Source: CAD feature listing. Evaluate the final solid. Frame: model axes, mm. Coordinates: 2 decimals unless noted, no trailing zeros. Order: outer loops, then holes, each group sorted by start corner. A loop starts at its lowest first (then second) coordinate and runs counter-clockwise, first axis right, second up.
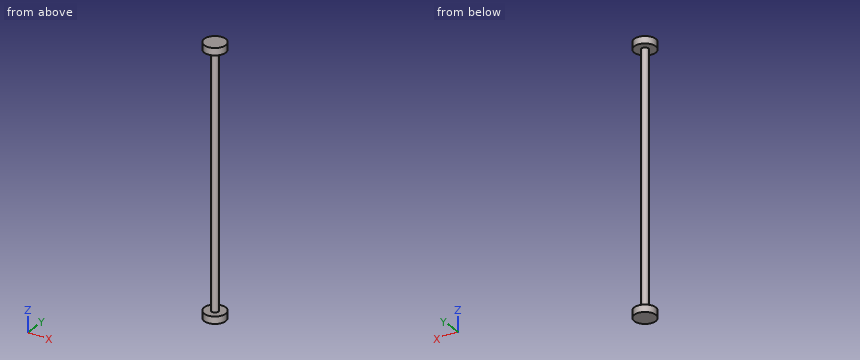
```python
from build123d import *

# Parameters (mm, degrees)
SKETCH1_R           = 12.7
BOSS_EXTRUDE2_DEPTH = 889
SKETCH4_R           = 38.1
BOSS_EXTRUDE4_DEPTH = 25.4
BOSS_EXTRUDE5_START = 25.4
SKETCH5_R           = 38.1
BOSS_EXTRUDE5_DEPTH = 25.4


with BuildPart() as part:
    # Sketch1 → Boss-Extrude2 (new body)
    with BuildSketch(Plane.XY):
        with Locations((-12.210402701, 19.442718147)):
            Circle(SKETCH1_R)
    extrude(amount=BOSS_EXTRUDE2_DEPTH)

    # Sketch4 → Boss-Extrude4 (add)
    with BuildSketch(Plane.XY.offset(889)):
        with Locations((-12.210402701, 19.442718147)):
            Circle(SKETCH4_R)
    extrude(amount=BOSS_EXTRUDE4_DEPTH)

    # Sketch5 → Boss-Extrude5 (add)
    with BuildSketch(Plane(origin=(0, 0, 0), x_dir=(-1, 0, 0), z_dir=(0, 0, -1)).offset(BOSS_EXTRUDE5_START)):
        with Locations(Location((12.210402701, 19.442718147, 0), (0, 0, 180))):
            Circle(SKETCH5_R)
    extrude(amount=-BOSS_EXTRUDE5_DEPTH)


solid = part.part
```
1. Section query A-A on x = 14. Return loops of the section in (y, z).
Findings:
outline: (-8.21, -25.4) - (47.09, -25.4) - (47.09, 0) - (-8.21, 0) - close; (-8.21, 889) - (47.09, 889) - (47.09, 914.4) - (-8.21, 914.4) - close
2. Section query C-C on z = 66. Return loops of the section in (x, y).
Findings:
outline: circle Ø25.4 at (-12.21, 19.44)
3. Ray query, line 1 (Z direction, x = 5, y = 15.5); line 2 (X direction, y = 19.5, z = 365); line 3 (Y direction, x = -19, z = 179.5). Return the intervals inside material, ascending.
Findings:
line 1: z = -25.4 to 0, 889 to 914.4
line 2: x = -24.91 to 0.49
line 3: y = 8.71 to 30.18
4. Pin query (flat end, axial travel): P1, Ø3, axis at x = -12.5, z = 614, coming from the +Y side; P2, Ø4, axis at y = 20.5, z = 311, coming from the +X side; P3, Ø3, axis at x = -22, z = 613.5, coming from the +Y side. Return the tip coordinate at first contact, or that it passes through.
Findings:
P1: stops at y = 32.14
P2: stops at x = 0.49
P3: stops at y = 29.06
5. Section query B-B on y = -10. Return loops of the section in (x, z), plus the area to 3 significant figures.
Findings:
outline: (-36.39, -25.4) - (11.97, -25.4) - (11.97, 0) - (-36.39, 0) - close; (-36.39, 889) - (11.97, 889) - (11.97, 914.4) - (-36.39, 914.4) - close
area: 2,460 mm2
